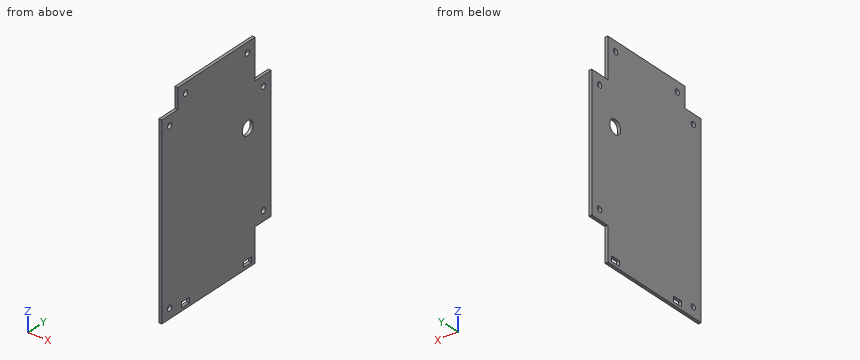
Autodesk Inventor part; units mm, degrees
ref_plane "YZ Plane" through (0, 0, 0) normal (1, 0, 0) x (0, 1, 0)
ref_plane "XZ Plane" through (0, 0, 0) normal (0, 1, 0) x (-1, 0, 0)
ref_plane "XY Plane" through (0, 0, 0) normal (0, 0, 1) x (1, 0, 0)
sketch "Sketch1" plane through (0, 0, 0) normal (1, 0, 0) x (0, 1, 0)
  line L0 (0, 0) -> (140, 0)
  line L1 (140, 0) -> (140, -210)
  line L2 (140, -210) -> (0, -210)
  line L3 (0, -210) -> (0, 0)
  dimension "d0" = 210
  dimension "d1" = 140
extrude "Extrusion1" add sketch "Sketch1" along normal blind 3
sketch "Sketch2" plane through (0, 0, 0) normal (-1, 0, 0) x (0, 0, 1)
  line L0 (0, 0) -> (-20.5, 0)
  line L1 (-20.5, 0) -> (-20.5, 20.5)
  line L2 (-20.5, 20.5) -> (0, 20.5)
  line L3 (0, 20.5) -> (0, 0)
  line L4 (-210, 140) -> (0, 140)
  line L5 (0, 140) -> (-40.5, 140)
  line L6 (-40.5, 140) -> (-40.5, 119.5)
  line L7 (-40.5, 119.5) -> (0, 119.5)
  line L8 (0, 119.5) -> (0, 140)
  line L9 (-210, 140) -> (-176, 140)
  line L10 (-176, 140) -> (-176, 119.5)
  line L11 (-176, 119.5) -> (-210, 119.5)
  line L12 (-210, 119.5) -> (-210, 140)
  point P0 (-176, 140)
  dimension "d4" = 20.5
  dimension "d5" = 20.5
  dimension "d6" = 40.5
  dimension "d7" = 20.5
  dimension "d8" = 34
extrude "Extrusion2" cut sketch "Sketch2" against normal blind 3
sketch "Sketch3" plane through (0, 0, 0) normal (-1, 0, 0) x (0, 0, 1)
  circle A0 centre (-10, 30.5) radius 2.75
  line L0 (-20.5, 20.5) -> (0, 20.5)
  line L1 (0, 119.5) -> (0, 20.5)
  circle A1 centre (-10, 109.5) radius 2.75
  circle A2 centre (-50.5, 130) radius 2.75
  circle A3 centre (-166, 130) radius 2.75
  circle A4 centre (-200, 10) radius 2.75
  circle A5 centre (-30.5, 10) radius 2.75
  line L2 (-20.5, 0) -> (-210, 0)
  line L3 (-20.5, 0) -> (-20.5, 20.5)
  line L4 (-210, 0) -> (-210, 119.5)
  line L5 (-176, 140) -> (-176, 119.5)
  line L6 (-176, 140) -> (-40.5, 140)
  line L7 (-40.5, 119.5) -> (-40.5, 140)
  line L8 (0, 119.5) -> (-40.5, 119.5)
  point P0 (0, 0)
  dimension "d11" = 5.5
  dimension "d12" = 10
  dimension "d13" = 10
  dimension "d14" = 10
  dimension "d15" = 10
  dimension "d16" = 10
  dimension "d17" = 10
  dimension "d18" = 10
  dimension "d19" = 10
  dimension "d20" = 10
  dimension "d21" = 10
  dimension "d22" = 10
  dimension "d23" = 10
  dimension "d24" = 5.5
  dimension "d25" = 5.5
  dimension "d26" = 5.5
  dimension "d27" = 5.5
  dimension "d28" = 5.5
extrude "Extrusion3" cut sketch "Sketch3" against normal blind 3
sketch "Sketch4" plane through (0, 0, 0) normal (-1, 0, 0) x (0, 0, 1)
  line L0 (-201.8, 25) -> (-207, 25)
  line L1 (-207, 25) -> (-207, 35.2)
  line L2 (-207, 35.2) -> (-201.8, 35.2)
  line L3 (-201.8, 35.2) -> (-201.8, 25)
  line L4 (-201.8, 104.8) -> (-207, 104.8)
  line L5 (-207, 104.8) -> (-207, 115)
  line L6 (-207, 115) -> (-201.8, 115)
  line L7 (-201.8, 115) -> (-201.8, 104.8)
  line L8 (-210, 0) -> (-210, 119.5)
  line L9 (-20.5, 0) -> (-210, 0)
  line L10 (-176, 119.5) -> (-210, 119.5)
  line L11 (-176, 140) -> (-40.5, 140)
  point P0 (0, 0)
  dimension "d31" = 3
  dimension "d32" = 25
  dimension "d34" = 10.2
  dimension "d35" = 10.2
  dimension "d36" = 5.2
  dimension "d37" = 25
extrude "Extrusion4" cut sketch "Sketch4" against normal blind 3
sketch "Sketch5" plane through (0, 0, 0) normal (-1, 0, 0) x (0, 0, 1)
  point P0 (0, 0)
sketch "Sketch6" plane through (0, 0, 0) normal (-1, 0, 0) x (0, 0, 1)
  circle A0 centre (-80, 110) radius 7
  line L0 (-176, 140) -> (-40.5, 140)
  line L1 (0, 119.5) -> (0, 20.5)
  line L2 (-176, 140) -> (-176, 119.5)
  point P0 (0, 0)
  dimension "d40" = 14
  dimension "d41" = 30
  dimension "d43" = 80
extrude "Extrusion5" cut sketch "Sketch6" against normal blind 3
equation "\"d5\" = d4"
equation "\"d13\" = d12"
equation "\"d14\" = d12"
equation "\"d15\" = d12"
equation "\"d16\" = d12"
equation "\"d17\" = d12"
equation "\"d18\" = d12"
equation "\"d19\" = d12"
equation "\"d20\" = d12"
equation "\"d21\" = d12"
equation "\"d22\" = d12"
equation "\"d23\" = d12"
equation "\"d24\" = d11"
equation "\"d25\" = d11"
equation "\"d26\" = d11"
equation "\"d27\" = d11"
equation "\"d28\" = d11"
properties part number "Steckerplatte_hint"
Geometry: final body of the model. Coordinates: model frame, mm. Round coordinates to 2 decimals unless told otherwise and drop trailing zeros. Loops run counter-clockwise (first coordinate to the right, second up) from the corner with the lowest first, then second, coordinate; pieces in that order, holes last. Notation, with made-up numbers: (46, -39.75) - (94, -39.75) arc R13 ccw to (94, -31.75) - close; hole circle Ø8 at (12, 19.25). An arc over 180 degrees is marked (long way). Write each question's results on one line, items separated by ' | '. Start each with the question number.
1) Line query: probe 1 along Z at (x, y) = (2.05, 31); probe 2 along Z at (x, y) = (1.3, 130); probe 3 along Y at (x, z) = (2.3, -31). Output: solid intervals per line, ascending. Write a range as [from, to].
2) First-contact query: P1, Ø4.5, axis at y = 10, z = -30.5, coming from the -X side (3 decimals); P2, Ø1.5, axis at x = 1.5, z = -203.5, coming from the +Y side. Flat tips, straight axial feed; report the tip coordinate or a pass-through.
3) Cut plane A-A on z = -80. Return loops of the section in (x, y), then the cut area to 3 significant figures.
4) Cut plane D-D on z = -30.5. Return loops of the section in (x, y).
5) Cut plane B-B on y = 10. Return loops of the section in (x, z), then the cut area to 4 significant figures.
6) Cut plane C-C on x = 0.5. Count the separate pieces of the cut face and the enclosed holes in it, then the cut area to 4 significant figures.
Verdict:
1) probe 1: z = [-210, -207], [-201.8, -12.7], [-7.3, 0] | probe 2: z = [-176, -168.75], [-163.25, -53.25], [-47.75, -40.5] | probe 3: y = [0, 7.3], [12.7, 119.5]
2) P1: passes through | P2: stops at y = 119.5
3) outline: (0, 0) - (3, 0) - (3, 103) - (0, 103) - close; (0, 117) - (3, 117) - (3, 140) - (0, 140) - close | area: 378 mm2
4) outline: (0, 0) - (3, 0) - (3, 7.25) - (0, 7.25) - close; (0, 12.75) - (3, 12.75) - (3, 119.5) - (0, 119.5) - close
5) outline: (0, -210) - (3, -210) - (3, -202.75) - (0, -202.75) - close; (0, -197.25) - (3, -197.25) - (3, -33.25) - (0, -33.25) - close; (0, -27.75) - (3, -27.75) - (3, -20.5) - (0, -20.5) - close | area: 535.5 mm2
6) separate pieces: 1 | enclosed holes: 9 | area: 27,050 mm2
